Work out the finished part from the listing and answer in its coordinate system (mm). Face numbers are marked on the shaded views. A direction names the side the tool comes from. Coordinates: 2 decimals unless noted, no trailing zeros. Write each loop counter-clockwise with the first axis right and the second up, starting at its lowest first coordinate (ties: lowest second). Pieces come first, ordered by that corner, then holes. Notation, with made-up numbers: (-7, 44) - (19, 44) arc R20 ccw to (19, 64) - close; hole circle Ø2 at (-10.5, 22.5). An arc over 180 degrees is marked (long way). Use one line per item in the form item = value. Start each with the question number.
Item 1: A cutting plane is placed at B-B (x = 7.5). Write down the section's boundary in (y, z).
Item 2: A cutting plane is placed at C-C (z = 5.5). Write down the section's boundary in (x, y), then the cut area to 3 significant figures.
Item 3: Determine the mould class of the marked faces 1, 2, 3 and 4 for opening direction X: released by +X, released by -X, zero draft, split by the parting line, or undercut.
Item 4: A cutting plane is placed at A-A (y = -5.5). Write down the section's boundary in (x, z).
Item 5: Consider probe 1 along Z at (x, y) = (-1, -8); probe 2 along X at (y, z) = (-6.25, -3.5); probe 3 along Z at (x, y) = (1, -5). Determine where each line is inside the solid, lowest interval first.
Item 6: For the marked faces 5 and 6, determine the directions among +Z, -Z, +X, -X, +Y, -Y from which every point of the face is accessible in a straight line to the end or side of a thin tool.
Item 7: Given pin 1 (2 mm diameter, centred on x = -2.5, y = -5, fed in from +Z); pin 2 (1 mm diameter, centred on y = -8.5, z = -9.5, fed in from +X); pin 3 (2 mm diameter, centred on x = 3.5, y = -5, fed in from -Z), each flat-ended and moving along its own axis, determine where each tip first touches the part or whether it passes through.
Item 8: A cutting plane is placed at D-D (z = 2.5). Write down the section's boundary in (x, y).
from build123d import *

# Parameters (mm, degrees)
F0_R     = 13.081
F1_DEPTH = 12.7


with BuildPart() as f1:
    # F0 (on Front) → F1 (new body)
    with BuildSketch(Plane.XZ):
        Circle(F0_R)
        with BuildLine():
            Line((-11.782692, -0.817253), (-8.666367, -0.76907))
            Line((-8.666367, -0.76907), (-8.552309, -8.146026))
            ThreePointArc((-8.552309, -8.146026), (-10.807673, -4.763815), (-11.782692, -0.817253))
        make_face(mode=Mode.SUBTRACT)
        with BuildLine():
            ThreePointArc((5.509203, -10.447411), (1.640638, -11.696496), (-2.422288, -11.559941))
            Line((-2.422288, -11.559941), (3.909314, -7.772686))
            Line((3.909314, -7.772686), (5.509203, -10.447411))
        make_face(mode=Mode.SUBTRACT)
        with BuildLine():
            Line((6.599107, -9.795484), (4.999218, -7.120759))
            Line((4.999218, -7.120759), (11.33082, -3.333504))
            ThreePointArc((11.33082, -3.333504), (9.529421, -6.977812), (6.599107, -9.795484))
        make_face(mode=Mode.SUBTRACT)
        with BuildLine():
            ThreePointArc((11.675552, 1.783592), (11.809589, 0.182593), (11.725112, -1.421785))
            Line((11.725112, -1.421785), (-4.29314, -11.003121))
            ThreePointArc((-4.29314, -11.003121), (-5.746664, -10.3187), (-7.093858, -9.443352))
            Line((-7.093858, -9.443352), (-7.382412, 9.219529))
            ThreePointArc((-7.382412, 9.219529), (-6.062924, 10.136107), (-4.631254, 10.865137))
            Line((-4.631254, 10.865137), (11.675552, 1.783592))
        make_face(mode=Mode.SUBTRACT)
        with BuildLine():
            ThreePointArc((-11.802325, 0.452596), (-10.949782, 4.427414), (-8.800058, 7.877734))
            Line((-8.800058, 7.877734), (-8.686, 0.500778))
            Line((-8.686, 0.500778), (-11.802325, 0.452596))
        make_face(mode=Mode.SUBTRACT)
        with BuildLine():
            Line((5.183584, 10.612737), (3.667149, 7.889829))
            Line((3.667149, 7.889829), (-2.778511, 11.47953))
            ThreePointArc((-2.778511, 11.47953), (1.278252, 11.741627), (5.183584, 10.612737))
        make_face(mode=Mode.SUBTRACT)
        with BuildLine():
            ThreePointArc((6.293122, 9.994816), (9.309144, 7.269082), (11.222347, 3.682207))
            Line((11.222347, 3.682207), (4.776687, 7.271908))
            Line((4.776687, 7.271908), (6.293122, 9.994816))
        make_face(mode=Mode.SUBTRACT)
    extrude(amount=F1_DEPTH)


solid = f1.part
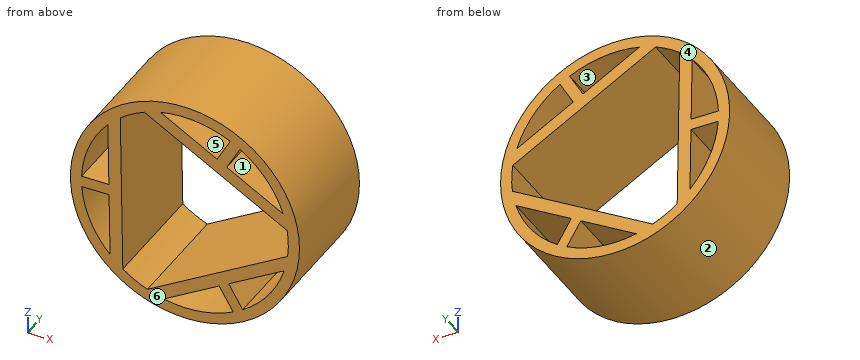
Answer:
q1.outline = (-12.7, -10.72) - (0, -10.72) - (0, -9.12) - (-12.7, -9.12) - close; (-12.7, -5.62) - (0, -5.62) - (0, -3.95) - (-12.7, -3.95) - close; (-12.7, 4.11) - (0, 4.11) - (0, 5.76) - (-12.7, 5.76) - close; (-12.7, 9.12) - (0, 9.12) - (0, 10.72) - (-12.7, 10.72) - close
q2.outline = (-11.87, -12.7) - (-10.45, -12.7) - (-10.45, 0) - (-11.87, 0) - close; (-8.76, -12.7) - (-7.32, -12.7) - (-7.32, 0) - (-8.76, 0) - close; (5, -12.7) - (7.96, -12.7) - (7.96, 0) - (5, 0) - close; (10.45, -12.7) - (11.87, -12.7) - (11.87, 0) - (10.45, 0) - close
q2.area = 91.8 mm²
q3.face_1 = undercut
q3.face_2 = split by the parting line
q3.face_3 = undercut
q3.face_4 = zero draft
q4.outline = circle Ø26.16 at (0, 0); hole (-11.8, 0.45) - (-8.69, 0.5) - (-8.8, 7.88) arc R11.81 ccw to start; hole (-11.78, -0.82) arc R11.81 ccw to (-8.55, -8.15) - (-8.67, -0.77) - close; hole (-7.38, 9.22) - (-7.09, -9.44) arc R11.81 ccw to (-4.29, -11) - (11.73, -1.42) arc R11.81 ccw to (11.68, 1.78) - (-4.63, 10.87) arc R11.81 ccw to start; hole (-2.78, 11.48) - (3.67, 7.89) - (5.18, 10.61) arc R11.81 ccw to start; hole (-2.42, -11.56) arc R11.81 ccw to (5.51, -10.45) - (3.91, -7.77) - close; hole (4.78, 7.27) - (11.22, 3.68) arc R11.81 ccw to (6.29, 9.99) - close; hole (5, -7.12) - (6.6, -9.8) arc R11.81 ccw to (11.33, -3.33) - close
q5.probe_1 = -13.04 to -11.77, -10.71 to -9.03, 8.84 to 10.49, 11.77 to 13.04
q5.probe_2 = -12.6 to -11.28, -8.62 to -7.19, 8.25 to 11.05, 11.28 to 12.6
q5.probe_3 = -13.04 to -11.77, -9.51 to -7.84, 7.73 to 9.38, 11.77 to 13.04
q6.face_5 = +Y, -Y
q6.face_6 = +Z, -Z, +X, -X, -Y
q7.pin_1 = 12.99
q7.pin_2 = 9.49
q7.pin_3 = -12.84
q8.outline = (-12.84, -12.7) - (-11.54, -12.7) - (-11.54, 0) - (-12.84, 0) - close; (-8.72, -12.7) - (-7.28, -12.7) - (-7.28, 0) - (-8.72, 0) - close; (10.39, -12.7) - (12.84, -12.7) - (12.84, 0) - (10.39, 0) - close
